Can you work these out from the drawing? Everything is in mm from the part's minimum corner. Coordinates: 2 decimals unless noted, no trailing zeros. Write each loop counter-clockwise with the first axis right and the second up, starting at its lowest first coordinate (ties: lowest second). Pieces come first, ordered by that corner, then holes. Notation, with made-up numbers: (60, 29.25) - (109, 29.25) arc R18 ccw to (109, 39.25) - close; hole circle Ø4 at (89, 62.25). An arc over 180 degrees is marked (long way). One line per question, with ' | ' between items. Start each with the question number.
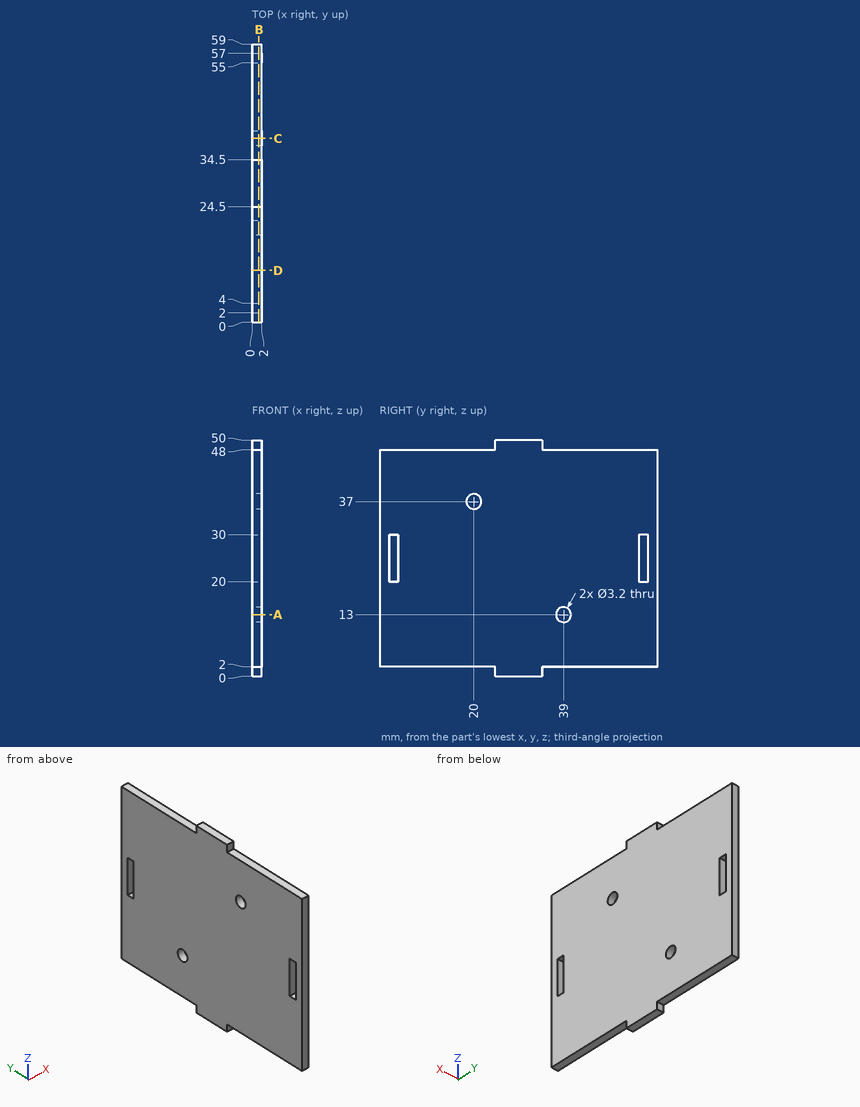
(1) If I drill on probe 1 along Y at (x, z) = (1.55, 24); probe 2 along Z at (x, y) = (1.5, 39); probe 3 along Z at (x, y) = (1.1, 20), over which ranges is the centre line in solid material (lowest first)?
(2) If we section it at D-D on y = 11: List the corners of the cut face in (x, z) for me, plus the area to 3 significant figures.
(3) If we section it at C-C on y = 39: List the corners of the cut face in (x, z) for me, plus the area to 3 significant figures.
(4) I'm going to push flat-ended pins straight in: pin 1 (1 mm diameter, centred on x = 0.5, y = 13, fed in from -Z); pin 2 (1 mm diameter, centred on x = 0.5, y = 7, fed in from +Z); pin 3 (1 mm diameter, centred on x = 1, z = 1, fed in from +Y). Where does each tip first touch, or does it pass through?
(5) If we section it at B-B on x = 1.4: List the corners of the cut face in (y, z) for me, plus the area to 3 significant figures.
(6) If we section it at A-A on z = 13: List the corners of the cut face in (x, y) for me, plus the area to 3 significant figures.
Values:
1) probe 1: 0 to 2, 4 to 55, 57 to 59 | probe 2: 2 to 11.4, 14.6 to 48 | probe 3: 2 to 35.4, 38.6 to 48
2) outline: (0, 2) - (2, 2) - (2, 48) - (0, 48) - close | area: 92.0 mm2
3) outline: (0, 2) - (2, 2) - (2, 11.4) - (0, 11.4) - close; (0, 14.6) - (2, 14.6) - (2, 48) - (0, 48) - close | area: 85.6 mm2
4) pin 1: z = 2 | pin 2: z = 48 | pin 3: y = 34.5
5) outline: (0, 2) - (24.5, 2) - (24.5, 0) - (34.5, 0) - (34.5, 2) - (59, 2) - (59, 48) - (34.5, 48) - (34.5, 50) - (24.5, 50) - (24.5, 48) - (0, 48) - close; hole (2, 20) - (4, 20) - (4, 30) - (2, 30) - close; hole circle Ø3.2 at (20, 37); hole circle Ø3.2 at (39, 13); hole (55, 20) - (57, 20) - (57, 30) - (55, 30) - close | area: 2,700 mm2
6) outline: (0, 0) - (2, 0) - (2, 37.4) - (0, 37.4) - close; (0, 40.6) - (2, 40.6) - (2, 59) - (0, 59) - close | area: 112 mm2
